```python
from build123d import *

# Parameters (mm, degrees)
F1_DEPTH = 1.3


with BuildPart() as f1:
    # F0 (on Right) → F1 (new body)
    with BuildSketch(Plane.YZ):
        with BuildLine():
            Line((-28.5022601296, 13.5822960047), (-30.0456807017, 12.1807558462))
            add(Edge.make_bspline(
                [(-30.0456807017, 12.1807558462), (-30.050324092, 12.1191925835), (-30.0456807017, 12.056948002)],
                knots=[0, 0, 0, 0.0248618931, 0.0248618931, 0.0248618931], degree=2, weights=[1, 0.9999227368, 1]))
            Line((-30.0456807017, 12.056948002), (-29.2544480902, 10.9238724842))
            add(Edge.make_bspline(
                [(-29.2544480902, 10.9238724842), (-6.4495956437, -6.866929483), (28.1840730012, 6.1202085385)],
                knots=[0.2427638345, 0.2427638345, 0.2427638345, 2.7999505323, 2.7999505323, 2.7999505323], degree=2, weights=[1, 0.2880625196, 1]))
            Line((28.1840730012, 6.1202085385), (30.0456807017, 7.7721911115))
            Line((30.0456807017, 7.7721911115), (29.5491017408, 8.6504284676))
            add(Edge.make_bspline(
                [(29.5491017408, 8.6504284676), (25.3237843176, 12.7552573017), (2.096655059, 14.7285637166), (-21.1304741996, 16.7018701315), (-28.5022601296, 13.5822960047)],
                knots=[3.3365042971, 3.3365042971, 3.3365042971, 4.6549863272, 4.6549863272, 5.9734683573, 5.9734683573, 5.9734683573], degree=2, weights=[1, 0.7904573504, 1, 0.7904573504, 1]))
        make_face()
        with BuildLine():
            Line((8.01217556, 46.7401072383), (-28.5022601296, 13.5822960047))
            add(Edge.make_bspline(
                [(29.5491017408, 8.6504284676), (25.3237843176, 12.7552573017), (2.096655059, 14.7285637166), (-21.1304741996, 16.7018701315), (-28.5022601296, 13.5822960047)],
                knots=[3.3365042971, 3.3365042971, 3.3365042971, 4.6549863272, 4.6549863272, 5.9734683573, 5.9734683573, 5.9734683573], degree=2, weights=[1, 0.7904573504, 1, 0.7904573504, 1]))
            Line((29.5491017408, 8.6504284676), (8.01217556, 46.7401072383))
        make_face()
        with BuildLine():
            add(Edge.make_bspline(
                [(-29.2544480902, 10.9238724842), (-6.4495956437, -6.866929483), (28.1840730012, 6.1202085385)],
                knots=[0.2427638345, 0.2427638345, 0.2427638345, 2.7999505323, 2.7999505323, 2.7999505323], degree=2, weights=[1, 0.2880625196, 1]))
            Line((-29.2544480902, 10.9238724842), (-5.2079111338, -23.5116928816))
            Line((-5.2079111338, -23.5116928816), (28.1840730012, 6.1202085385))
        make_face()
    extrude(amount=F1_DEPTH)


solid = f1.part
```
Input: part model. Units: mm. Frame: model coordinates. Round coordinates to 2 decimals unless told otherwise and drop trailing zeros. Order: outer loops, then holes, each group sorted by start corner. A loop starts at its lowest first (then second) coordinate and runs counter-clockwise, first axis right, second up. Notation, with made-up numbers: (-31, 43) - (0, 43) arc R20 ccw to (0, 75) - close; hole circle Ø10 at (-39.5, 12.5). An arc over 180 degrees is marked (long way). One line per question, with ' | ' between items. Start each with the question number.
1) Cut plane B-B, the plane y = -20. Return the cut outline in (x, z), then the cut area to 3 significant figures.
2) Cut plane A-A, the plane z = 4. Return the cut outline in (x, y), then the cut area to 3 significant figures.
3) Ray query, probe 1 along Y at (x, z) = (0.3, 21.5); probe 2 along Z at (x, y) = (0.9, 4.5); probe 3 along Z at (x, y) = (0.9, -23.5). Return the intervals inside material, ascending.
Worked out:
1) outline: (0, -2.33) - (1.3, -2.33) - (1.3, 21.3) - (0, 21.3) - close | area: 30.7 mm^2
2) outline: (0, -24.42) - (1.3, -24.42) - (1.3, 25.79) - (0, 25.79) - close | area: 65.3 mm^2
3) probe 1: y = -19.78 to 22.28 | probe 2: z = -14.9 to 43.55 | probe 3: z = 2.68 to 18.12
